The listing builds one solid part. Answer for the finished solid, in the listing's coordinates (mm). Face numbers are marked on the shaded views. Give positions to 0.01 mm unless a question says otherwise; leave off trailing zeros. Order: outer loops, then holes, each group sorted by start corner. A loop starts at its lowest first (then second) coordinate and runs counter-clockwise, first axis right, second up. Notation, with made-up numbers: (15.25, 29.25) - (68.25, 29.25) arc R22 cw to (68.25, 66.25) - close; hole circle Ø6 at (-6, 87.5). An arc over 180 degrees is marked (long way). Answer as a JSON object with one key per item and string values. Group by question number.
Q1. A cutting plane is placed at C-C, the plane z = 22.4. Give the vertices of the cut face in (x, y).
Q2. A cutting plane is placed at D-D, the plane y = 3. Give the vertices of the cut face in (x, z), and give its area (3 significant figures).
Q3. A cutting plane is placed at A-A, the plane x = 0.5. Give the vertices of the cut face in (y, z), and give its area (3 significant figures).
Q4. A cutting plane is placed at B-B, the plane y = -5.25. Give the vertices of the cut face in (x, z), and give its area (3 significant figures).
Q5. Given pin 1 (1 mm diameter, centred on x = -1, y = 0, fed in from -Z); pin 2 (1.5 mm diameter, centred on x = 0.5, z = 13, fed in from +Y), each flat-ended and moving along its own axis, determine where each tip first touches the part or whether it passes through.
Q6. Consider line 1 (Z direction, x = 1.3, y = -4); line 2 (Z direction, x = 0.2, y = -5); line 3 (Y direction, x = 0.7, z = 22.4). Determine where each line is inside the solid, lowest interval first.
Q7. The mould has two halves that part along Z. Classify the marked faces 1, 2 and 3: released by +Z, released by -Z, zero draft, split by the parting line, or undercut.
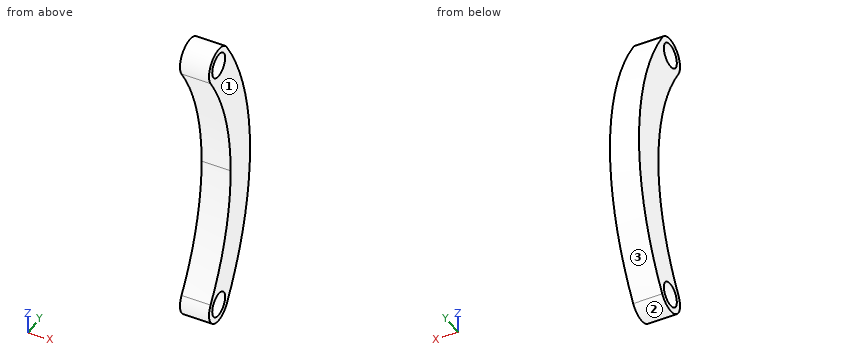
from build123d import *

# Parameters (mm, degrees)
BOSS_EXTRUDE1_DEPTH = 2.399999953
SKETCH2_R           = 2
CUT_EXTRUDE1_DEPTH  = 4.8


with BuildPart() as part:
    # Sketch1 → Boss-Extrude1 (new body, symmetric)
    with BuildSketch(Plane(origin=(0, 0, 0), x_dir=(0, 0, -1), z_dir=(1, 0, 0))):
        with BuildLine():
            ThreePointArc((0, 0), (10.830584713, -1.585060066), (20.752730266, -6.207289856))
            ThreePointArc((20.752730266, -6.207289856), (24.907289856, -5.347269734), (24.047269734, -1.192710144))
            ThreePointArc((24.047269734, -1.192710144), (12.549962758, 4.163308324), (0, 6))
            ThreePointArc((0, 6), (-12.549962758, 4.163308324), (-24.047269734, -1.192710144))
            ThreePointArc((-24.047269734, -1.192710144), (-24.907289856, -5.347269734), (-20.752730266, -6.207289856))
            ThreePointArc((-20.752730266, -6.207289856), (-10.830584713, -1.585060066), (0, 0))
        make_face()
    extrude(amount=BOSS_EXTRUDE1_DEPTH, both=True)

    # Sketch2 → Cut-Extrude1 (cut)
    with BuildSketch(Plane(origin=(2.399999953, 0, 0), x_dir=(0, 0, -1), z_dir=(1, 0, 0))):
        with Locations((-22.4, -3.7)):
            Circle(SKETCH2_R)
        with Locations((22.4, -3.7)):
            Circle(SKETCH2_R)
    extrude(amount=-CUT_EXTRUDE1_DEPTH, mode=Mode.SUBTRACT)


solid = part.part
Reply:
{
 "1": {"outline": "(-2.4, -6.7) - (2.4, -6.7) - (2.4, -5.7) - (-2.4, -5.7) - close; (-2.4, -1.7) - (2.4, -1.7) - (2.4, -0.16) - (-2.4, -0.16) - close"},
 "2": {"outline": "(-2.4, -15.93) - (2.4, -15.93) - (2.4, 15.93) - (-2.4, 15.93) - close", "area": "153 mm^2"},
 "3": {"outline": "(-6.21, -20.75) arc R3 ccw to (-1.19, -24.05) arc R43.79 ccw to (-1.19, 24.05) arc R3 ccw to (-6.21, 20.75) arc R37.79 cw to start; hole circle Ø4 at (-3.7, -22.4); hole circle Ø4 at (-3.7, 22.4)", "area": "288 mm^2"},
 "4": {"outline": "(-2.4, -24.97) - (2.4, -24.97) - (2.4, -23.66) - (-2.4, -23.66) - close; (-2.4, -21.14) - (2.4, -21.14) - (2.4, -19.22) - (-2.4, -19.22) - close; (-2.4, 19.22) - (2.4, 19.22) - (2.4, 21.14) - (-2.4, 21.14) - close; (-2.4, 23.66) - (2.4, 23.66) - (2.4, 24.97) - (-2.4, 24.97) - close", "area": "31.0 mm^2"},
 "5": {"pin 1": "stops at z = -22.96", "pin 2": "stops at y = 4.25"},
 "6": {"line 1": "z = -25.38 to -24.38, -20.42 to -16.92, 16.92 to 20.42, 24.38 to 25.38", "line 2": "z = -25.1 to -23.92, -20.88 to -18.79, 18.79 to 20.88, 23.92 to 25.1", "line 3": "y = -6.7 to -5.7, -1.7 to -0.16"},
 "7": {"face 1": "zero draft", "face 2": "undercut", "face 3": "split by the parting line"}
}
